Can you work these out from the model? Positions are in its coordinate system, mm. Face numbers are marked on the shaded views. A direction names the side the tool comes from. Give positions to 0.01 mm unless a question says otherwise; leave off trailing zeros. Loops run counter-clockwise (first coordinate to the right, second up) from the corner with the lowest first, then second, coordinate; pieces in that order, holes last. Notation, with made-up numbers: (64.25, 48.25) -> (118.25, 48.25) arc R12 cw to (118.25, 63.25) -> close; hole circle Ø9 at (64, 14). An arc over 180 degrees is marked (long way). Use CSV: the item, a comma, the result in double quotes.
from build123d import *

# Parameters (mm, degrees)
SKETCH1_W           = 50.8
SKETCH1_H           = 86.242198053
BOSS_EXTRUDE1_DEPTH = 6.35
SKETCH1_3_W         = 50.8
SKETCH1_3_H         = 6.35
BOSS_EXTRUDE2_DEPTH = 38.1
SKETCH2_W           = 50.8
SKETCH2_H           = 86.242198053
SKETCH2_H_2         = 6.35
BOSS_EXTRUDE4_DEPTH = 6.35


with BuildPart() as part:
    # Sketch1 → Boss-Extrude1 (new body)
    with BuildSketch(Plane.XY):
        with Locations((-965.320655189, 591.828631034)):
            Rectangle(SKETCH1_W, SKETCH1_H)
        Polygon((-969.04135584, 603.19973006), (-972.707530049, 609.54973006), (-969.04135584, 615.89973006), (-961.709007421, 615.89973006), (-958.042833212, 609.54973006), (-961.709007421, 603.19973006), align=None, mode=Mode.SUBTRACT)
    extrude(amount=BOSS_EXTRUDE1_DEPTH)

    # Sketch1_3 → Boss-Extrude2 (add)
    with BuildSketch(Plane.XY):
        with Locations((-965.320655189, 545.532532007)):
            Rectangle(SKETCH1_3_W, SKETCH1_3_H)
    extrude(amount=BOSS_EXTRUDE2_DEPTH)

    # Sketch2 → Boss-Extrude4 (add)
    # profile 1 of 2: a face of its own
    with BuildSketch(Plane.XY.offset(38.1)):
        with Locations((-965.320655189, 591.828631034)):
            Rectangle(SKETCH2_W, SKETCH2_H)
        Polygon((-958.042833212, 609.54973006), (-961.709007421, 603.19973006), (-969.04135584, 603.19973006), (-972.707530049, 609.54973006), (-969.04135584, 615.89973006), (-961.709007421, 615.89973006), align=None, mode=Mode.SUBTRACT)
    # profile 2 of 2: a face of its own
    with BuildSketch(Plane.XY.offset(38.1)):
        with Locations((-965.320655189, 545.532532007)):
            Rectangle(SKETCH2_W, SKETCH2_H_2)
    extrude(amount=BOSS_EXTRUDE4_DEPTH)


solid = part.part
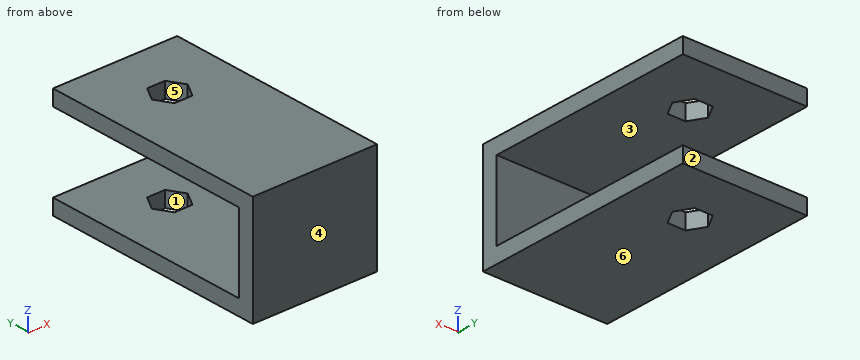
(1) If we section it at C-C, the plane x = -948.5: Write out the boundary of the cut face in (y, z), then the cut area to 3 significant figures.
Answer sheet:
outline,"(542.36, 0) -> (634.95, 0) -> (634.95, 6.35) -> (548.71, 6.35) -> (548.71, 38.1) -> (634.95, 38.1) -> (634.95, 44.45) -> (542.36, 44.45) -> close"
area,"1,380 mm2"
(2) If we section it at B-B, the plane y = 553.5: Write out the boundary of the cut face in (x, z).
Answer sheet:
outline,"(-990.72, 0) -> (-939.92, 0) -> (-939.92, 6.35) -> (-990.72, 6.35) -> close; (-990.72, 38.1) -> (-939.92, 38.1) -> (-939.92, 44.45) -> (-990.72, 44.45) -> close"
(3) If we section it at D-D, the plane y = 605: Write out the boundary of the cut face in (x, z), then the cut area to 3 significant figures.
Answer sheet:
outline,"(-990.72, 0) -> (-970.08, 0) -> (-970.08, 6.35) -> (-990.72, 6.35) -> close; (-990.72, 38.1) -> (-970.08, 38.1) -> (-970.08, 44.45) -> (-990.72, 44.45) -> close; (-960.67, 0) -> (-939.92, 0) -> (-939.92, 6.35) -> (-960.67, 6.35) -> close; (-960.67, 38.1) -> (-939.92, 38.1) -> (-939.92, 44.45) -> (-960.67, 44.45) -> close"
area,"526 mm2"
(4) Will this pin go through, and if not, where does the flat tip stop? pin 1 Ø9.5 at (x, z) = (-966.5, 28) entering from +Y.
Answer sheet:
pin 1,"stops at y = 548.71"
(5) If I drill on L1, parallel to Z at x = -974, y = 584; L2, parallel to Y at x = -976, z = 23.5, over which ranges is the centre line in solid material (lowest first)? Write a range as from..to.
Answer sheet:
L1,"z = 0..6.35, 38.1..44.45"
L2,"y = 542.36..548.71"
(6) Which directions (+Z, -Z, +X, -X, +Y, -Y) give clear straight access to the entire face, cutting with the end or side of a thin tool? Please do the marked faces 1, 2 and 3.
Answer sheet:
face 1,"+Z, -Z"
face 2,"+Z, -Z, +X, -X, +Y"
face 3,"+X, -X, +Y"
(7) If we section it at A-A, the plane x = -965.5: Write out the boundary of the cut face in (y, z).
Answer sheet:
outline,"(542.36, 0) -> (603.2, 0) -> (603.2, 6.35) -> (548.71, 6.35) -> (548.71, 38.1) -> (603.2, 38.1) -> (603.2, 44.45) -> (542.36, 44.45) -> close; (615.9, 0) -> (634.95, 0) -> (634.95, 6.35) -> (615.9, 6.35) -> close; (615.9, 38.1) -> (634.95, 38.1) -> (634.95, 44.45) -> (615.9, 44.45) -> close"
(8) We'd pull the mould along Y, two halves only. Please class the marked faces 4, 5 and 6: released by +Y, released by -Y, zero draft, split by the parting line, or undercut.
Answer sheet:
face 4,"released by -Y"
face 5,"undercut"
face 6,"zero draft"
